from build123d import *

# Parameters (mm, degrees)
SKETCH_1_W                 = 120
SKETCH_1_H                 = 68
EXTRUDE_1_DEPTH            = 5
SKETCH_2_W                 = 120
SKETCH_2_H                 = 2.5
EXTRUDE_2_DEPTH            = 5
CUT_EXTRUDE_1_REACH        = 71.145
SKETCH_3_W                 = 114
SKETCH_3_H                 = 10
SKETCH_4_W                 = 5
SKETCH_4_H                 = 26
EXTRUDE_3_DEPTH            = 20
SKETCH_5_W                 = 13
SKETCH_5_H                 = 26
EXTRUDE_4_DEPTH            = 5
CUT_EXTRUDE_2_REACH        = 77.206
SKETCH_6_W                 = 8
SKETCH_6_H                 = 2
HOLE_WIZARD_M3_1_OUTLINE_R = 1.7
HOLE_WIZARD_M3_1_DEPTH     = 5


# Read off the part's stored shape, not the designer's step: M3 すきま穴1
with BuildPart() as part:
    # ｽｹｯﾁ1 → ﾎﾞｽ - 押し出し1 (new body)
    with BuildSketch(Plane.XY):
        Rectangle(SKETCH_1_W, SKETCH_1_H)
    extrude(amount=EXTRUDE_1_DEPTH)

    # ｽｹｯﾁ2 → ﾎﾞｽ - 押し出し2 (add)
    with BuildSketch(Plane(origin=(0, 0, 0), x_dir=(-1, 0, 0), z_dir=(0, 0, -1))):
        with Locations((0, 32.75)):
            Rectangle(SKETCH_2_W, SKETCH_2_H)
        with Locations((0, 14.25)):
            Rectangle(SKETCH_2_W, SKETCH_2_H)
        with Locations((0, -14.25)):
            Rectangle(SKETCH_2_W, SKETCH_2_H)
        with Locations((0, -32.75)):
            Rectangle(SKETCH_2_W, SKETCH_2_H)
    extrude(amount=EXTRUDE_2_DEPTH)

    # ｽｹｯﾁ3 → ｶｯﾄ - 押し出し1 (cut, up to next)
    with BuildSketch(Plane(origin=(0, 0, 0), x_dir=(-1, 0, 0), z_dir=(0, 0, -1)), mode=Mode.PRIVATE) as cut_extrude_1_sk1:
        with Locations((0, 23.5)):
            Rectangle(SKETCH_3_W, SKETCH_3_H)
    cut_extrude_1_tool1 = extrude(cut_extrude_1_sk1.sketch, amount=-CUT_EXTRUDE_1_REACH, mode=Mode.PRIVATE) & part.part
    # ｽｹｯﾁ3 → ｶｯﾄ - 押し出し1 (cut, up to next)
    with BuildSketch(Plane(origin=(0, 0, 0), x_dir=(-1, 0, 0), z_dir=(0, 0, -1)), mode=Mode.PRIVATE) as cut_extrude_1_sk2:
        with Locations((0, -23.5)):
            Rectangle(SKETCH_3_W, SKETCH_3_H)
    cut_extrude_1_tool2 = extrude(cut_extrude_1_sk2.sketch, amount=-CUT_EXTRUDE_1_REACH, mode=Mode.PRIVATE) & part.part
    add(cut_extrude_1_tool1.solids().sort_by_distance((0, 23.5, 0))[0], mode=Mode.SUBTRACT)
    add(cut_extrude_1_tool2.solids().sort_by_distance((0, -23.5, 0))[0], mode=Mode.SUBTRACT)

    # ｽｹｯﾁ4 → ﾎﾞｽ - 押し出し3 (add)
    with BuildSketch(Plane(origin=(0, 0, 0), x_dir=(-1, 0, 0), z_dir=(0, 0, -1))):
        with Locations((-43, 0)):
            Rectangle(SKETCH_4_W, SKETCH_4_H)
        with Locations((43, 0)):
            Rectangle(SKETCH_4_W, SKETCH_4_H)
    extrude(amount=EXTRUDE_3_DEPTH)

    # ｽｹｯﾁ5 → ﾎﾞｽ - 押し出し4 (add)
    with BuildSketch(Plane(origin=(0, 0, -20), x_dir=(-1, 0, 0), z_dir=(0, 0, -1))):
        with Locations((-39, 0)):
            Rectangle(SKETCH_5_W, SKETCH_5_H)
        with Locations((39, 0)):
            Rectangle(SKETCH_5_W, SKETCH_5_H)
    extrude(amount=EXTRUDE_4_DEPTH)

    # ｽｹｯﾁ6 → ｶｯﾄ - 押し出し2 (cut, up to next)
    with BuildSketch(Plane(origin=(0, 0, -25), x_dir=(-1, 0, 0), z_dir=(0, 0, -1)), mode=Mode.PRIVATE) as cut_extrude_2_sk1:
        with Locations((-36.5, 0)):
            Rectangle(SKETCH_6_W, SKETCH_6_H)
    cut_extrude_2_tool1 = extrude(cut_extrude_2_sk1.sketch, amount=-CUT_EXTRUDE_2_REACH, mode=Mode.PRIVATE) & part.part
    # ｽｹｯﾁ6 → ｶｯﾄ - 押し出し2 (cut, up to next)
    with BuildSketch(Plane(origin=(0, 0, -25), x_dir=(-1, 0, 0), z_dir=(0, 0, -1)), mode=Mode.PRIVATE) as cut_extrude_2_sk2:
        with Locations((36.5, 0)):
            Rectangle(SKETCH_6_W, SKETCH_6_H)
    cut_extrude_2_tool2 = extrude(cut_extrude_2_sk2.sketch, amount=-CUT_EXTRUDE_2_REACH, mode=Mode.PRIVATE) & part.part
    add(cut_extrude_2_tool1.solids().sort_by_distance((36.5, 0, -25))[0], mode=Mode.SUBTRACT)
    add(cut_extrude_2_tool2.solids().sort_by_distance((-36.5, 0, -25))[0], mode=Mode.SUBTRACT)

    # M3 すきま穴1 outline → M3 すきま穴1 (cut)
    with BuildSketch(Plane.XY):
        with Locations((0, 10)):
            Circle(HOLE_WIZARD_M3_1_OUTLINE_R)
        with Locations((-37.5, 0)):
            Circle(HOLE_WIZARD_M3_1_OUTLINE_R)
    extrude(amount=HOLE_WIZARD_M3_1_DEPTH, mode=Mode.SUBTRACT)

    # Hole Wizard M3 _1 2 outline → Hole Wizard M3 _1 2 (revolve, cut)
    with BuildSketch(Plane(origin=(-37.5, 0, 0), x_dir=(1, 0, 0), z_dir=(0, -1, 0))):
        Polygon((1.7, -24.97124079), (1.7, -20), (0, -20), (0, -25.000000133), (1.725000116, -25.000000133), align=None)
    revolve(axis=Axis((-37.5, 0, 0), (0, 0, 1)), mode=Mode.SUBTRACT)

    # Hole Wizard M3 _1 3 outline → Hole Wizard M3 _1 3 (revolve, cut)
    with BuildSketch(Plane(origin=(-37.5, 10, 0), x_dir=(1, 0, 0), z_dir=(0, -1, 0))):
        Polygon((1.7, -24.97124079), (1.7, -20), (0, -20), (0, -25), (1.725, -25), align=None)
    revolve(axis=Axis((-37.5, 10, 0), (0, 0, 1)), mode=Mode.SUBTRACT)

    # Hole Wizard M3 _1 4 outline → Hole Wizard M3 _1 4 (revolve, cut)
    with BuildSketch(Plane(origin=(37.5, -10, 0), x_dir=(1, 0, 0), z_dir=(0, -1, 0))):
        Polygon((1.7, -24.97124079), (1.7, -20), (0, -20), (0, -25), (1.725, -25), align=None)
    revolve(axis=Axis((37.5, -10, 0), (0, 0, 1)), mode=Mode.SUBTRACT)

    # Hole Wizard M3 _1 5 outline → Hole Wizard M3 _1 5 (revolve, cut)
    with BuildSketch(Plane(origin=(-37.5, -10, 0), x_dir=(1, 0, 0), z_dir=(0, -1, 0))):
        Polygon((1.7, -24.97124079), (1.7, -20), (0, -20), (0, -25), (1.725, -25), align=None)
    revolve(axis=Axis((-37.5, -10, 0), (0, 0, 1)), mode=Mode.SUBTRACT)

    # Hole Wizard M3 _1 6 outline → Hole Wizard M3 _1 6 (revolve, cut)
    with BuildSketch(Plane(origin=(37.5, 10, 0), x_dir=(1, 0, 0), z_dir=(0, -1, 0))):
        Polygon((1.7, -24.97124079), (1.7, -20), (0, -20), (0, -25), (1.725, -25), align=None)
    revolve(axis=Axis((37.5, 10, 0), (0, 0, 1)), mode=Mode.SUBTRACT)


solid = part.part
Can you work these out from the model? Positions are in its coordinate system, mm. A direction names the side the tool comes from. Round coordinates to 2 decimals unless told otherwise and drop trailing zeros. Loops run counter-clockwise (first coordinate to the right, second up) from the corner with the lowest first, then second, coordinate; pieces in that order, holes last. Notation, with made-up numbers: (6, 87.25) - (53, 87.25) arc R15 cw to (53, 96.25) - close; hole circle Ø2 at (-20.75, 9). An arc over 180 degrees is marked (long way). Write item = value, one per line. Start each with the question number.
(1) If I drill on probe 1 along Y at (x, z) = (37.5, -21.8); probe 2 along Y at (x, z) = (20, 3.5); probe 3 along Y at (x, z) = (46, -3.5), over which ranges is the centre line in solid material (lowest first)? Write a range as [from, to].
(2) If we mould it in two halves opening along Y, with no side actions, what happens to faces 1 (the face through (-40.5, 0, -10)), 2 (the face through (42, 13, -17)), 3 (the face through (1, 14, -5))? For each: released by +Y, released by -Y, zero draft, split by the parting line, or undercut.
(3) If we section it at B-B (y = 10): Give the number of separate pieces and of enclosed holes in the cut face, and give its area (3 significant figures).
(4) For faces 4 (the face through (-53, 0, 0)), 5 (the face through (37, -7, -20)), 6 (the face through (32.5, 7, -22)), 7 (the face through (1, 15.5, -2)), which set-ups out of +Z, -Z, +X, -X, +Y, -Y let a thin tool reach every point of the face, with its end or its side?
(5) If we section it at C-C (z = -9.5): Please give me the cut outline in (x, y), and give its area (3 significant figures).
(6) If we section it at A-A (x = 0): Please give me the cut outline in (y, z).
(7) For P1, Ø14.5, axis at x = -42, z = -17, coming from the -Y side; P2, Ø8, axis at x = -34, z = -21.5, coming from the +Y side; P3, Ø3, axis at x = -27, y = 32, coming from the -Z side; P4, Ø12, axis at x = 47, y = -24.5, coming from the +Z side, each with a flat end and sliding along its axis, tell me the tip position at first contact or that it passes through.
(8) If we section it at D-D (y = -10): Please give me the cut outline in (x, z) (3 decimals).
Ans:
q1.probe_1 = [-13, -11.7], [-8.3, -1], [1, 8.3], [11.7, 13]
q1.probe_2 = [-34, -28.5], [-18.5, 18.5], [28.5, 34]
q1.probe_3 = [-34, -31.5], [-15.5, -13], [13, 15.5], [31.5, 34]
q2.face_1 = undercut
q2.face_2 = released by +Y
q2.face_3 = zero draft
q3.separate_pieces = 4
q3.enclosed_holes = 0
q3.area = 879 mm²
q4.face_4 = -Z, -X
q4.face_5 = +Y, -Y
q4.face_6 = -Z, +Y, -Y
q4.face_7 = -Z, +X, -X
q5.outline = (-45.5, -13) - (-40.5, -13) - (-40.5, 13) - (-45.5, 13) - close; (40.5, -13) - (45.5, -13) - (45.5, 13) - (40.5, 13) - close
q5.area = 260 mm²
q6.outline = (-34, -5) - (-31.5, -5) - (-31.5, 0) - (-28.5, 0) - (-28.5, 5) - (-34, 5) - close; (-18.5, 0) - (-15.5, 0) - (-15.5, -5) - (-13, -5) - (-13, 0) - (8.3, 0) - (8.3, 5) - (-18.5, 5) - close; (11.7, 0) - (13, 0) - (13, -5) - (15.5, -5) - (15.5, 0) - (18.5, 0) - (18.5, 5) - (11.7, 5) - close; (28.5, 0) - (31.5, 0) - (31.5, -5) - (34, -5) - (34, 5) - (28.5, 5) - close
q7.P1 = -13
q7.P2 = 13
q7.P3 = -5
q7.P4 = 5
q8.outline = (-60, 0) - (-45.5, 0) - (-45.5, -25) - (-39.225, -25) - (-39.2, -24.971) - (-39.2, -20) - (-40.5, -20) - (-40.5, 0) - (40.5, 0) - (40.5, -20) - (39.2, -20) - (39.2, -24.971) - (39.225, -25) - (45.5, -25) - (45.5, 0) - (60, 0) - (60, 5) - (-60, 5) - close; (-35.8, -24.971) - (-35.775, -25) - (-32.5, -25) - (-32.5, -20) - (-35.8, -20) - close; (32.5, -25) - (35.775, -25) - (35.8, -24.971) - (35.8, -20) - (32.5, -20) - close
